```python
from build123d import *

# Parameters (mm, degrees)
SKETCH1_W               = 107.95
SKETCH1_H               = 146.05
BOSS_EXTRUDE1_DEPTH     = 2.54
SKETCH13_W              = 25.4
SKETCH13_H              = 25.4
BOSS_EXTRUDE4_DEPTH     = 19.431
SKETCH2_R               = 3.302
CUT_EXTRUDE1_DEPTH      = 93.862882849
FILLET1_R               = 12.7
CUT_EXTRUDE13_DEPTH     = 5.08
SKETCH15_R              = 6.35
BOSS_EXTRUDE5_DEPTH     = 11.811
SKETCH23_R              = 2.25
CUT_EXTRUDE14_DEPTH     = 92.934228941
SKETCH24_R              = 4
CUT_EXTRUDE15_DEPTH     = 3.81
MIRROR2_COPY_1_SKETCH_R = 2.25
MIRROR2_COPY_1_DEPTH    = 92.934228941
MIRROR2_COPY_2_SKETCH_R = 4
MIRROR2_COPY_2_DEPTH    = 3.81
FILLET3_R               = 12.7
FILLET4_R               = 1.016


with BuildPart() as part:
    # Sketch1 → Boss-Extrude1 (new body)
    with BuildSketch(Plane(origin=(0, 0, 0), x_dir=(1, 0, 0), z_dir=(0, 1, 0))):
        Rectangle(SKETCH1_W, SKETCH1_H)
    extrude(amount=-BOSS_EXTRUDE1_DEPTH)

    # Sketch13 → Boss-Extrude4 (add)
    with BuildSketch(Plane(origin=(0, 0, 0), x_dir=(1, 0, 0), z_dir=(0, 1, 0))):
        with Locations((41.275, -60.325)):
            Rectangle(SKETCH13_W, SKETCH13_H)
        with Locations((-41.275, -60.325)):
            Rectangle(SKETCH13_W, SKETCH13_H)
        with Locations((-41.275, 60.325)):
            Rectangle(SKETCH13_W, SKETCH13_H)
        with Locations((41.275, 60.325)):
            Rectangle(SKETCH13_W, SKETCH13_H)
    extrude(amount=-BOSS_EXTRUDE4_DEPTH)

    # Sketch2 → Cut-Extrude1 (cut, through all)
    with BuildSketch(Plane(origin=(0, 0, 0), x_dir=(1, 0, 0), z_dir=(0, 1, 0))):
        with Locations(Location((-41.275, 60.325, 0), (0, 0, 270))):
            Circle(SKETCH2_R)
        with Locations(Location((41.275, 60.325, 0), (0, 0, 90))):
            Circle(SKETCH2_R)
        with Locations(Location((41.275, -60.325, 0), (0, 0, 270))):
            Circle(SKETCH2_R)
        with Locations(Location((-41.275, -60.325, 0), (0, 0, 90))):
            Circle(SKETCH2_R)
    extrude(amount=-CUT_EXTRUDE1_DEPTH, mode=Mode.SUBTRACT)

    # Fillet1
    fillet1_edges = [part.edges().sort_by_distance(p)[0] for p in [
        (53.975, -9.7155, 73.025),
        (-53.975, -9.7155, 73.025),
        (-53.975, -9.7155, -73.025),
        (53.975, -9.7155, -73.025),
    ]]
    fillet(fillet1_edges, radius=FILLET1_R)

    # Sketch14 → Cut-Extrude13 (cut)
    with BuildSketch(Plane.XZ.offset(19.431)):
        Polygon((20.692003582, -28.674172721), (6.35, -45.983487389), (139.336989519, -156.172707277), (153.678993101, -138.863392609), align=None)
        Polygon((-20.692003582, -28.674172721), (-6.35, -45.983487389), (-139.336989519, -156.172707277), (-153.678993101, -138.863392609), align=None)
        Polygon((-153.678993101, 138.863392609), (-20.692003582, 28.674172721), (-6.35, 45.983487389), (-139.336989519, 156.172707277), align=None)
        Polygon((20.692003582, 28.674172721), (6.35, 45.983487389), (139.336989519, 156.172707277), (153.678993101, 138.863392609), align=None)
    extrude(amount=-CUT_EXTRUDE13_DEPTH, mode=Mode.SUBTRACT)

    # Sketch15 → Boss-Extrude5 (add)
    with BuildSketch(Plane(origin=(0, 0, 0), x_dir=(1, 0, 0), z_dir=(0, 1, 0))):
        with Locations((-41.275, 60.325)):
            Circle(SKETCH15_R)
        with Locations((41.275, 60.325)):
            Circle(SKETCH15_R)
        with Locations((-41.275, -60.325)):
            Circle(SKETCH15_R)
        with Locations((41.275, -60.325)):
            Circle(SKETCH15_R)
    extrude(amount=-BOSS_EXTRUDE5_DEPTH)

    # Sketch23 → Cut-Extrude14 (cut, through all)
    with BuildSketch(Plane.XZ.offset(14.351)):
        with Locations(Location((-41.275, -60.325, 0), (0, 0, 270))):
            Circle(SKETCH23_R)
    cut_extrude14 = extrude(amount=-CUT_EXTRUDE14_DEPTH, mode=Mode.SUBTRACT)

    # Sketch24 → Cut-Extrude15 (cut)
    with BuildSketch(Plane(origin=(0, 0, 0), x_dir=(1, 0, 0), z_dir=(0, 1, 0))):
        with Locations(Location((-41.275, 60.325, 0), (0, 0, 270))):
            Circle(SKETCH24_R)
    cut_extrude15 = extrude(amount=-CUT_EXTRUDE15_DEPTH, mode=Mode.SUBTRACT)

    # Mirror1: Cut-Extrude14, Cut-Extrude15 across plane
    add(cut_extrude14.mirror(Plane.XY), mode=Mode.SUBTRACT)
    add(cut_extrude15.mirror(Plane.XY), mode=Mode.SUBTRACT)

    # Mirror2: Cut-Extrude14, Cut-Extrude15 across plane
    add(cut_extrude14.mirror(Plane(origin=(0, 0, 0), x_dir=(0, 0, 1), z_dir=(1, 0, 0))), mode=Mode.SUBTRACT)
    add(cut_extrude15.mirror(Plane(origin=(0, 0, 0), x_dir=(0, 0, 1), z_dir=(1, 0, 0))), mode=Mode.SUBTRACT)

    # Mirror2 copy 1 sketch → Mirror2 copy 1 (cut, through all)
    with BuildSketch(Plane(origin=(0, -14.351, 0), x_dir=(-1, 0, 0), z_dir=(0, -1, 0))):
        with Locations(Location((-41.275, -60.325, 0), (0, 0, 270))):
            Circle(MIRROR2_COPY_1_SKETCH_R)
    extrude(amount=-MIRROR2_COPY_1_DEPTH, mode=Mode.SUBTRACT)

    # Mirror2 copy 2 sketch → Mirror2 copy 2 (cut)
    with BuildSketch(Plane(origin=(0, 0, 0), x_dir=(-1, 0, 0), z_dir=(0, 1, 0))):
        with Locations(Location((-41.275, 60.325, 0), (0, 0, 270))):
            Circle(MIRROR2_COPY_2_SKETCH_R)
    extrude(amount=-MIRROR2_COPY_2_DEPTH, mode=Mode.SUBTRACT)

    # Fillet3
    fillet3_edges = [part.edges().sort_by_distance(p)[0] for p in [
        (28.575, -8.4455, -47.625),
        (-28.575, -8.4455, -47.625),
        (-28.575, -8.4455, 47.625),
        (28.575, -8.4455, 47.625),
    ]]
    fillet(fillet3_edges, radius=FILLET3_R)

    # Fillet4
    fillet4_edges = [part.edges().sort_by_distance(p)[0] for p in [
        (41.275, -14.351, -57.023),
        (-41.275, -14.351, -63.627),
        (-41.275, -14.351, 63.627),
        (41.275, -14.351, 57.023),
    ]]
    fillet(fillet4_edges, radius=FILLET4_R)


solid = part.part
```
Source: CAD feature listing. Evaluate the final solid. Frame: model axes, mm. A direction names the side the tool comes from. Round coordinates to 2 decimals unless told otherwise and drop trailing zeros. Order: outer loops, then holes, each group sorted by start corner. A loop starts at its lowest first (then second) coordinate and runs counter-clockwise, first axis right, second up. Notation, with made-up numbers: (-12.5, -28) -> (3.5, -28) arc R12 cw to (3.5, -5) -> close; hole circle Ø11 at (24.25, 63.25). An arc over 180 degrees is marked (long way). Use CSV: the item, a comma, the result in double quotes.
(1) Section C-C on z = 0. Return the cut outline in (x, y) (3 decimals).
Report:
outline,"(-53.975, -2.54) -> (53.975, -2.54) -> (53.975, 0) -> (-53.975, 0) -> close"
(2) Section A-A on y = -8.25. Return the cut outline in (x, z) (3 decimals).
Report:
outline,"(-53.975, -60.325) arc R12.7 ccw to (-41.275, -73.025) -> (-28.575, -73.025) -> (-28.575, -60.325) arc R12.7 ccw to (-41.275, -47.625) -> (-53.975, -47.625) -> close; (-53.975, 47.625) -> (-41.275, 47.625) arc R12.7 ccw to (-28.575, 60.325) -> (-28.575, 73.025) -> (-41.275, 73.025) arc R12.7 ccw to (-53.975, 60.325) -> close; (28.575, -73.025) -> (41.275, -73.025) arc R12.7 ccw to (53.975, -60.325) -> (53.975, -47.625) -> (41.275, -47.625) arc R12.7 ccw to (28.575, -60.325) -> close; (28.575, 60.325) arc R12.7 ccw to (41.275, 47.625) -> (53.975, 47.625) -> (53.975, 60.325) arc R12.7 ccw to (41.275, 73.025) -> (28.575, 73.025) -> close; hole circle Ø4.5 at (-41.275, -60.325); hole circle Ø4.5 at (-41.275, 60.325); hole circle Ø4.5 at (41.275, -60.325); hole circle Ø4.5 at (41.275, 60.325)"
(3) Section D-D on x = 33.5. Return the cut outline in (y, z) (3 decimals).
Report:
outline,"(-19.431, -73.025) -> (0, -73.025) -> (0, 73.025) -> (-19.431, 73.025) -> (-19.431, 68.479) -> (-14.351, 68.479) -> (-14.351, 50.283) -> (-2.54, 50.283) -> (-2.54, -50.283) -> (-14.351, -50.283) -> (-14.351, -68.479) -> (-19.431, -68.479) -> close"
(4) First-contact query: pin 1 Ø5 at (y, z) = (-4, -4.5) entering from -X (3 decimals); pin 2 Ø4 at (x, z) = (40, -61.5) entering from +Y; pin 3 Ø10 at (x, y) = (-46.5, -9.5) entering from +Z; pin 4 Ø10.5 at (x, z) = (41.275, -60.325) entering from -Y. Flat tips, straight axial feed; report the tip coordinate or a pass-through.
Report:
pin 1,"x = -53.975"
pin 2,"y = -3.81"
pin 3,"z = 73.02"
pin 4,"y = -14.35"
(5) Section B-B on x = -17. Return the cut outline in (y, z) (3 decimals), and give its area (3 significant figures).
Report:
outline,"(-2.54, -73.025) -> (0, -73.025) -> (0, 73.025) -> (-2.54, 73.025) -> close"
area,"371 mm^2"
(6) Ray query, L1, parallel to Z at x = 41.5, y = -1.5; L2, parallel to X at y = -4, z = -61 (3 decimals); L3, parallel to X at y = -3.75, z = 63.5 (3 decimals). Return the intervals inside material, ascending.
Report:
L1,"-73.02 to -64.32, -56.33 to 56.33, 64.32 to 73.02"
L2,"-53.957 to -43.421, -39.129 to -28.575, 28.575 to 39.129, 43.421 to 53.957"
L3,"-53.572 to -43.708, -38.842 to -28.575, 28.575 to 38.842, 43.708 to 53.572"
(7) Access query for faces 4 (the face through (32.39, -8.53, 51.25)), 5 (the face through (41.1, -1.88, -64.32)), 6 (the face through (48, -11, -47.625)), 7 (the face through (28.575, -11, -67)). Directions: +Z, -Z, +X, -X, +Y, -Y. A direction counts if a zero-diameter tool reaches every point of the face in a straight line with its end or side. Return the directions, or none.
Report:
face 4,"-Y"
face 5,"+Y"
face 6,"+X, -X, -Y"
face 7,"+Z, -Z, -Y"
(8) Pull-direction query (X, two-part tool) for faces 1 (the face through (-3, -2, 73.025)), 2 (the face through (48.842, -16.927, -51.999)), 3 (the face through (50.35, -7.28, 69.21)); classes: +X half, -X half, draft (parallel to the pull), parting line (faces both ways), or undercut.
Report:
face 1,"draft"
face 2,"undercut"
face 3,"+X half"
